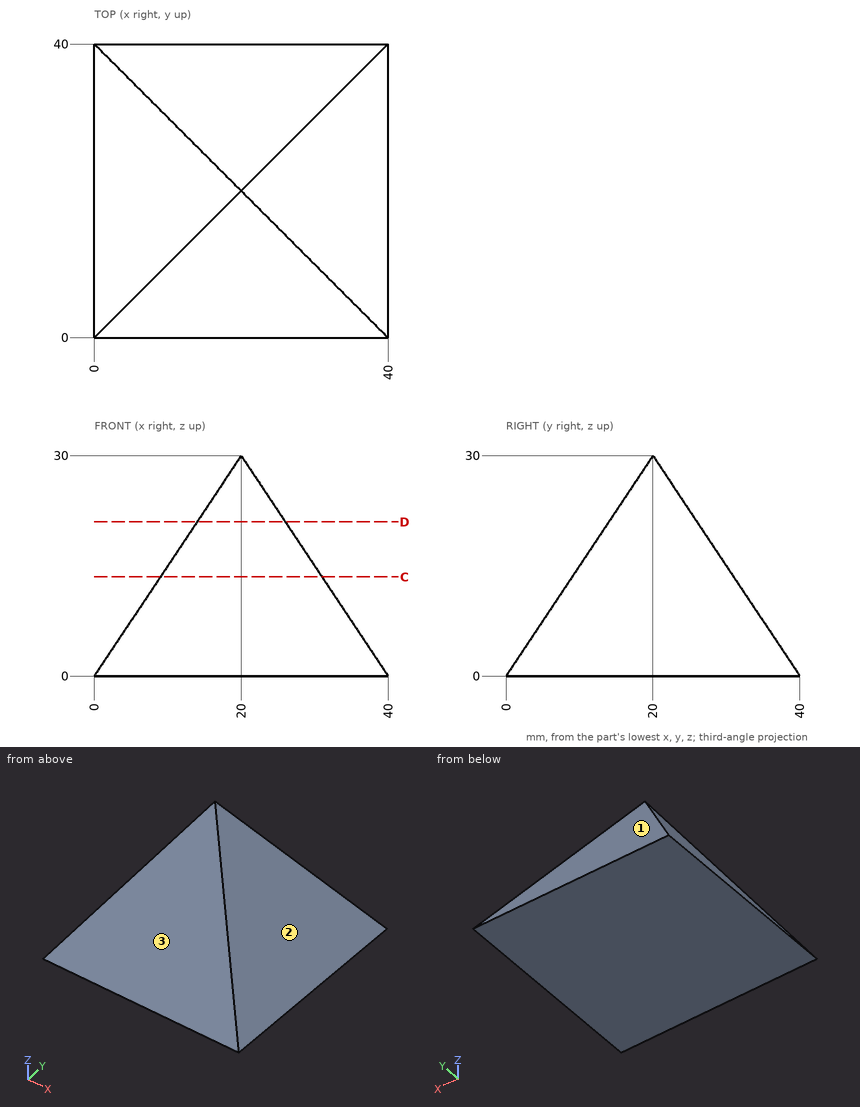
Input: dimensioned drawing with shaded views. Units: mm. Origin: part minimum x, y, z. Give positions to 0.01 mm unless a question says otherwise; leave off trailing zeros. Write each loop counter-clockwise with the first axis right and the second up, starting at its lowest first coordinate (ties: lowest second). Pieces come first, ordered by that corner, then holes. Notation, with made-up numbers: (36.25, -30) - (91.25, -30) arc R7 ccw to (91.25, -17) - close; hole circle Ø6 at (45, 63). An arc over 180 degrees is marked (long way). Write item = value, one per line. Start each with the question number.
1) Draft query along Y for the marked faces 1, 2 and 3. Return one class per face: pulls with the +Y half, pulls with the -Y half, needs draft (parallel to the pull), parting line crosses it, or undercut.
2) Cut plane D-D (z = 21). Return loops of the section in (x, y), and give its area (3 significant figures).
3) Pin query (flat end, axial travel): pin 1 (6 mm diameter, centred on x = 5, y = 5, fed in from +Z); pin 2 (2 mm diameter, centred on x = 23, z = 3.5, fed in from +Y); pin 3 (1.5 mm diameter, centred on x = 30, y = 17.5, fed in from +Z) (3 decimals); pin 4 (10 mm diameter, centred on y = 5.5, z = 18.5, fed in from -X). Return the tip coordinate at first contact, or that it passes through.
4) Cut plane C-C (z = 13.5). Return loops of the section in (x, y).
5) Material intervals for L1, parallel to Z at x = 5, y = 35.5; L2, parallel to Z at x = 10.5, y = 36; L3, parallel to X at y = 23, z = 6.75, sorted ascending. Write a range as [from, to].
Answers follow:
q1.face_1 = pulls with the +Y half
q1.face_2 = needs draft
q1.face_3 = pulls with the -Y half
q2.outline = (14, 14) - (26, 14) - (26, 26) - (14, 26) - close
q2.area = 144 mm^2
q3.pin_1 = 10.68
q3.pin_2 = 38.33
q3.pin_3 = 16.125
q3.pin_4 = through
q4.outline = (9, 9) - (31, 9) - (31, 31) - (9, 31) - close
q5.L1 = [0, 6.75]
q5.L2 = [0, 6]
q5.L3 = [4.5, 35.5]
